from build123d import *

# Parameters (mm, degrees)
SKETCH1_W           = 31.8
SKETCH1_H           = 84
BOSS_EXTRUDE1_DEPTH = 2
SKETCH2_W           = 27.8
SKETCH2_H           = 79.9
BOSS_EXTRUDE2_DEPTH = 0.001
SKETCH3_W           = 5
SKETCH3_H           = 10
BOSS_EXTRUDE3_DEPTH = 9
CUT_EXTRUDE1_DEPTH  = 3
SKETCH5_R           = 1.6
CUT_EXTRUDE2_DEPTH  = 2


with BuildPart() as part:
    # Sketch1 → Boss-Extrude1 (new body)
    with BuildSketch(Plane.XY):
        Rectangle(SKETCH1_W, SKETCH1_H)
    extrude(amount=BOSS_EXTRUDE1_DEPTH)

    # Sketch2 → Boss-Extrude2 (add)
    with BuildSketch(Plane(origin=(0, 0, 0), x_dir=(-1, 0, 0), z_dir=(0, 0, -1))):
        Rectangle(SKETCH2_W, SKETCH2_H)
    extrude(amount=BOSS_EXTRUDE2_DEPTH)

    # Sketch3 → Boss-Extrude3 (add)
    with BuildSketch(Plane(origin=(0, 0, 0), x_dir=(-1, 0, 0), z_dir=(0, 0, -1))):
        with Locations((-11.4, 0)):
            Rectangle(SKETCH3_W, SKETCH3_H)
    extrude(amount=BOSS_EXTRUDE3_DEPTH)

    # Sketch4 → Cut-Extrude1 (cut)
    with BuildSketch(Plane.ZY.offset(-8.9)):
        Polygon((-2.41228676, 2.75), (-5.58771324, 2.75), (-7.175426481, 0), (-5.58771324, -2.75), (-2.41228676, -2.75), (-0.824573519, 0), align=None)
    extrude(amount=-CUT_EXTRUDE1_DEPTH, mode=Mode.SUBTRACT)

    # Sketch5 → Cut-Extrude2 (cut)
    with BuildSketch(Plane.ZY.offset(-11.9)):
        with Locations((-4, 0)):
            Circle(SKETCH5_R)
    extrude(amount=-CUT_EXTRUDE2_DEPTH, mode=Mode.SUBTRACT)


solid = part.part
Geometry check sheet. Reference: the model listing, model coordinates, mm. A direction names the side the tool comes from. Round coordinates to 2 decimals unless told otherwise and drop trailing zeros. Loops run counter-clockwise (first coordinate to the right, second up) from the corner with the lowest first, then second, coordinate; pieces in that order, holes last.
Item 1: Cross-section at A-A on z = -4. Record the boundary of the cut face in (x, y), then the cut area to 3 significant figures.
Item 2: Thickness scan on line 1 (Y direction, x = 13.1, z = -4); line 2 (Y direction, x = 12, z = -7); line 3 (Z direction, x = -4.5, y = -20). Record the ranges inside material, lowest first.
Item 3: Mould release check, pull along Y, two halves, no side actions. Record for faces 4 (the flat face through (-14.2, 3.3, 0)), 5 (the flat face through (10.38, -1.36, -6.39)), 6 (the flat face through (10.38, 1.36, -1.61)), 7 (the flat face through (0, 42, 1)): pulls with the +Y half, pulls with the -Y half, needs draft (parallel to the pull), parting line crosses it, or undercut.
Item 4: Gauge pin test, flat ends, axial feed: pin 1 (3 mm diameter, centred on y = -1, z = -3.5, fed in from -X); pin 2 (2.5 mm diameter, centred on x = 11, z = -4.5, fed in from +Y); pin 3 (2 mm diameter, centred on y = -25.5, z = -0.5, fed in from +X); pin 4 (4 mm diameter, centred on y = 0, z = -4, fed in from +X). Record the tip position at first contact, or that the pin passes through.
Item 5: Cross-section at D-D on z = -8. Record the boundary of the cut face in (x, y), then the cut area to 3 significant figures.
Item 6: Access from +Z, -Z, +X, -X, +Y, -Y to the whole of each face (thin tool, end or side, straight path). Record for faces 1 (the flat face through (8.9, -0.1, -7.4)), 2 (the flat face through (13.9, 0, -6)), 3 (the flat face through (11.9, 1.3, -2.6)).
Answer sheet:
1. outline: (8.9, -5) - (13.9, -5) - (13.9, -1.6) - (11.9, -1.6) - (11.9, -2.75) - (8.9, -2.75) - close; (8.9, 2.75) - (11.9, 2.75) - (11.9, 1.6) - (13.9, 1.6) - (13.9, 5) - (8.9, 5) - close
1. area: 27.1 mm2
2. line 1: y = -5 to -1.6, 1.6 to 5
2. line 2: y = -5 to 5
2. line 3: z = 0 to 2
3. face 4: needs draft
3. face 5: undercut
3. face 6: undercut
3. face 7: pulls with the +Y half
4. pin 1: stops at x = 11.9
4. pin 2: stops at y = 5
4. pin 3: stops at x = 15.9
4. pin 4: stops at x = 13.9
5. outline: (8.9, -5) - (13.9, -5) - (13.9, 5) - (8.9, 5) - close
5. area: 50.0 mm2
6. face 1: -Z, -X, +Y, -Y
6. face 2: -Z, +X, +Y, -Y
6. face 3: -X
